```python
from build123d import *

# Parameters (mm, degrees)
BOSS_EXTRUDE1_DEPTH = 5
SKETCH3_W           = 5
SKETCH3_H           = 5
CUT_EXTRUDE1_DEPTH  = 5
SKETCH4_R           = 7.5
CUT_EXTRUDE2_DEPTH  = 10


with BuildPart() as part:
    # Sketch2 → Boss-Extrude1 (new body)
    with BuildSketch(Plane.XY):
        Polygon((-61.802768985, 20.649350649), (-11.802768985, 20.649350649), (17, 73.283944775), (17, -19.350649351), (0, -19.350649351), (0, -64.350649351), (-40, -64.350649351), (-40, -19.350649351), (-61.802768985, -19.350649351), (-101.802768985, -19.350649351), align=None)
    extrude(amount=BOSS_EXTRUDE1_DEPTH)

    # Sketch3 → Cut-Extrude1 (cut)
    with BuildSketch(Plane.XY.offset(5)):
        with Locations((-54.302768985, 15.149350649)):
            Rectangle(SKETCH3_W, SKETCH3_H)
        with Locations((-19.302768985, 15.149350649)):
            Rectangle(SKETCH3_W, SKETCH3_H)
    extrude(amount=-CUT_EXTRUDE1_DEPTH, mode=Mode.SUBTRACT)

    # Sketch4 → Cut-Extrude2 (cut)
    with BuildSketch(Plane.XY.offset(5)):
        with Locations((-20, -44.350649351)):
            Circle(SKETCH4_R)
    extrude(amount=-CUT_EXTRUDE2_DEPTH, mode=Mode.SUBTRACT)


solid = part.part
```
Source: CAD feature listing. Evaluate the final solid. Frame: model axes, mm. A direction names the side the tool comes from. Give positions to 0.01 mm unless a question says otherwise; leave off trailing zeros. Write each loop counter-clockwise with the first axis right and the second up, starting at its lowest first coordinate (ties: lowest second). Pieces come first, ordered by that corner, then holes.
1. Material intervals for line 1 along Y through (x, z) = (-20, 1.6); line 2 along X through (y, z) = (-54.5, 3.1); line 3 along X through (y, z) = (-51, 0.3), sorted ascending.
2. Pull-direction query (Y, two-part tool) for faces 1 (the face through (-37, 20.649, 2)), 2 (the face through (-51.803, 15, 3)), 3 (the face through (17, 28, 2)); classes: +Y half, -Y half, draft (parallel to the pull), parting line (faces both ways), or undercut.
3. Section query D-D (y = 8). Return the cut outline in (x, z).
4. Section query A-A (x = -20). Return the cut outline in (y, z).
5. Section query C-C (x = -49). Return the cut outline in (y, z).
6. First-contact query: pin 1 (1 mm diameter, centred on y = -37.5, z = 3.5, fed in from +X); pin 2 (2.5 mm diameter, centred on y = 15.5, z = 3.5, fed in from -X); pin 3 (3 mm diameter, centred on x = -55, z = 3, fed in from +Y). Flat tips, straight axial feed; report the tip coordinate or a pass-through.
7. Section query B-B (z = 2.9). Return the cut outline in (x, y), then the cut area to 3 significant figures.
8. Access query for faces 4 (the face through (-54, 17.649, 3)), 5 (the face through (-40, -42, 2)), 6 (the face through (0, -42, 2)). Directions: +Z, -Z, +X, -X, +Y, -Y. A direction counts if a zero-diameter tool reaches every point of the face in a straight line with its end or side. Return the directions, or none.
Output values:
1. line 1: y = -64.35 to -51.85, -36.85 to 12.65, 17.65 to 20.65
1. line 2: x = -40 to 0
1. line 3: x = -40 to -23.47, -16.53 to 0
2. face 1: +Y half
2. face 2: undercut
2. face 3: draft
3. outline: (-74.45, 0) - (17, 0) - (17, 5) - (-74.45, 5) - close
4. outline: (-64.35, 0) - (-51.85, 0) - (-51.85, 5) - (-64.35, 5) - close; (-36.85, 0) - (12.65, 0) - (12.65, 5) - (-36.85, 5) - close; (17.65, 0) - (20.65, 0) - (20.65, 5) - (17.65, 5) - close
5. outline: (-19.35, 0) - (20.65, 0) - (20.65, 5) - (-19.35, 5) - close
6. pin 1: stops at x = 0
6. pin 2: stops at x = -68.2
6. pin 3: stops at y = 20.65
7. outline: (-101.8, -19.35) - (-40, -19.35) - (-40, -64.35) - (0, -64.35) - (0, -19.35) - (17, -19.35) - (17, 73.28) - (-11.8, 20.65) - (-61.8, 20.65) - close; hole (-56.8, 12.65) - (-51.8, 12.65) - (-51.8, 17.65) - (-56.8, 17.65) - close; hole circle Ø15 at (-20, -44.35); hole (-21.8, 12.65) - (-16.8, 12.65) - (-16.8, 17.65) - (-21.8, 17.65) - close
7. area: 6,280 mm2
8. face 4: +Z, -Z
8. face 5: +Z, -Z, -X, -Y
8. face 6: +Z, -Z, +X, -Y
